from build123d import *

# Parameters (mm, degrees)
TEST_BOX_START     = -10
TEST_BOX_PROFILE_W = 20
TEST_BOX_PROFILE_H = 20
TEST_BOX_DEPTH     = 20
TEST_CUT_START     = -12
TEST_CUT_PROFILE_R = 2
TEST_CUT_DEPTH     = 24


with BuildPart() as part:
    # Test_box_Profile → Test_box (new body)
    with BuildSketch(Plane.XY.offset(TEST_BOX_START)):
        Rectangle(TEST_BOX_PROFILE_W, TEST_BOX_PROFILE_H)
    extrude(amount=TEST_BOX_DEPTH)

    # Test_cut_Profile → Test_cut (cut)
    with BuildSketch(Plane.XY.offset(TEST_CUT_START)):
        with Locations(Location((0, 0, 0), (0, 0, 180))):
            Circle(TEST_CUT_PROFILE_R)
    extrude(amount=TEST_CUT_DEPTH, mode=Mode.SUBTRACT)


solid = part.part
Model file for the job. Use its own axes, mm. Give positions to 0.01 mm unless a question says otherwise; leave off trailing zeros. Loops run counter-clockwise (first coordinate to the right, second up) from the corner with the lowest first, then second, coordinate; pieces in that order, holes last.
1) Pull direction X, two halves, no side cores. Call faces 1 (the flat face through (-0.1, 2.4, 10)), 2 (the flat face through (-10, 0, 0)), 3 (the cylindrical face through (0, 2, 0)): +X half, -X half, draft (parallel to the pull), parting line (faces both ways), or undercut.
2) Wall check: line 1 (Y direction, x = 0, z = -3); line 2 (Y direction, x = 0.5, z = -4.5); line 3 (X direction, y = -1.5, z = -3.75). Give the ranges that are in metal, low to high.
3) Saw through at A-A (y = 0). Write the cut outline in (x, z).
4) Flat gauge pin, fed straight in: pin 1 Ø5 at (x, y) = (0, -1.5) entering from +Z. Where does the tip first touch, or does it go through?
5) Saw through at C-C (z = 3.75). Write the cut outline in (x, y).
Answer block:
1. face 1: draft
1. face 2: -X half
1. face 3: undercut
2. line 1: y = -10 to -2, 2 to 10
2. line 2: y = -10 to -1.94, 1.94 to 10
2. line 3: x = -10 to -1.32, 1.32 to 10
3. outline: (-10, -10) - (-2, -10) - (-2, 10) - (-10, 10) - close; (2, -10) - (10, -10) - (10, 10) - (2, 10) - close
4. pin 1: stops at z = 10
5. outline: (-10, -10) - (10, -10) - (10, 10) - (-10, 10) - close; hole circle Ø4 at (0, 0)
